The listing builds one solid part. Answer for the finished solid, in the listing's coordinates (mm). Face numbers are marked on the shaded views. A direction names the side the tool comes from. Give positions to 0.01 mm unless a question says otherwise; leave off trailing zeros. Loops run counter-clockwise (first coordinate to the right, second up) from the corner with the lowest first, then second, coordinate; pieces in that order, holes last.
Item 1: Each of these flat-tipped pins is pushed along its axis until it touches: pin 1 Ø1.5 at (x, y) = (4.5, 3.5) entering from -Z; pin 2 Ø1.5 at (x, y) = (-7.5, 2.5) entering from -Z; pin 3 Ø1.5 at (x, y) = (8, 6) entering from +Z. Where does it stop, or does it pass through?
Item 2: The mould has two halves that part along X. Classify the marked faces 3, 4, 5 and 6: pulls with the +X half, pulls with the -X half, needs draft (parallel to the pull), parting line crosses it, or undercut.
Item 3: Consider line 1 along Z through (x, y) = (4, 6); line 2 along Z through (x, y) = (2, 1.25); line 3 along X through (y, z) = (6.75, 6). Determine where each line is inside the solid, lowest interval first.
Item 4: Section D-D, the plane x = -12.5 is taken. Give the vertices of the cut face in (y, z).
Item 5: Section C-C, the plane x = 5 is taken. Give the vertices of the cut face in (y, z), and give its area (3 significant figures).
Item 6: Section B-B, the plane z = 0 is taken. Give the vertices of the cut face in (x, y), and give its area (3 significant figures).
Item 7: A tool of negligible diameter and unlimited length cuts with its end or side. For the marked faces 1 and 2, from which of +Z, -Z, +X, -X, +Y, -Y can it reach the whole face along a straight path? Write none if from no direction.
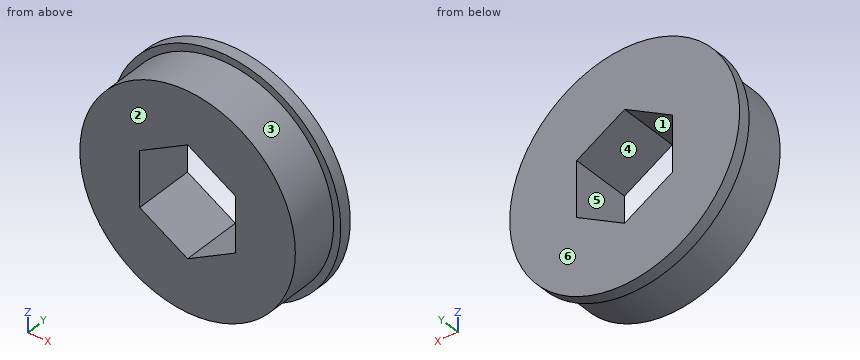
from build123d import *

# Parameters (mm, degrees)
SKETCH1_R           = 14.2875
BOSS_EXTRUDE1_DEPTH = 6.35
SKETCH2_R           = 15.24
BOSS_EXTRUDE2_DEPTH = 1.5748


with BuildPart() as part:
    # Sketch1 → Boss-Extrude1 (new body)
    with BuildSketch(Plane(origin=(0, 0, 0), x_dir=(1, 0, 0), z_dir=(0, 1, 0))):
        with Locations(Location((0, 0, 0), (0, 0, 270))):
            Circle(SKETCH1_R)
        Polygon((0, -7.332348419), (6.35, -3.666174209), (6.35, 3.666174209), (0, 7.332348419), (-6.35, 3.666174209), (-6.35, -3.666174209), align=None, mode=Mode.SUBTRACT)
    extrude(amount=BOSS_EXTRUDE1_DEPTH)

    # Sketch2 → Boss-Extrude2 (add)
    with BuildSketch(Plane(origin=(0, 6.35, 0), x_dir=(1, 0, 0), z_dir=(0, 1, 0))):
        with Locations(Location((0, 0, 0), (0, 0, 270))):
            Circle(SKETCH2_R)
        Polygon((0, 7.332348419), (-6.35, 3.666174209), (-6.35, -3.666174209), (0, -7.332348419), (6.35, -3.666174209), (6.35, 3.666174209), align=None, mode=Mode.SUBTRACT)
    extrude(amount=BOSS_EXTRUDE2_DEPTH)


solid = part.part
Worked answers:
1. pin 1: stops at z = -13.79
1. pin 2: stops at z = -12.59
1. pin 3: stops at z = 13.36
2. face 3: parting line crosses it
2. face 4: undercut
2. face 5: undercut
2. face 6: needs draft
3. line 1: z = -13.72 to -5.02, 5.02 to 13.72
3. line 2: z = -14.15 to -6.18, 6.18 to 14.15
3. line 3: x = -14.01 to -2.31, 2.31 to 14.01
4. outline: (0, -6.92) - (6.35, -6.92) - (6.35, -8.72) - (7.92, -8.72) - (7.92, 8.72) - (6.35, 8.72) - (6.35, 6.92) - (0, 6.92) - close
5. outline: (0, -13.38) - (6.35, -13.38) - (6.35, -14.4) - (7.92, -14.4) - (7.92, -4.45) - (0, -4.45) - close; (0, 4.45) - (7.92, 4.45) - (7.92, 14.4) - (6.35, 14.4) - (6.35, 13.38) - (0, 13.38) - close
5. area: 145 mm2
6. outline: (-15.24, 6.35) - (-14.29, 6.35) - (-14.29, 0) - (-6.35, 0) - (-6.35, 7.92) - (-15.24, 7.92) - close; (6.35, 0) - (14.29, 0) - (14.29, 6.35) - (15.24, 6.35) - (15.24, 7.92) - (6.35, 7.92) - close
6. area: 129 mm2
7. face 1: +Y, -Y
7. face 2: +Z, -Z, +X, -X, -Y
